Geometry check sheet. Reference: the model listing, model coordinates, mm. Round coordinates to 2 decimals unless told otherwise and drop trailing zeros. Order: outer loops, then holes, each group sorted by start corner. A loop starts at its lowest first (then second) coordinate and runs counter-clockwise, first axis right, second up. Notation, with made-up numbers: M 88.25,19.5 L 92.25,19.5 A27 cw 92.25,35.5 Z; hole C -19,89 d11. An arc over 180 degrees is marked long. Answer as a JSON object with one key per item and string values. Group by question number.
```python
from build123d import *

# Parameters (mm, degrees)
SKETCH_W            = 603
SKETCH_H            = 451
SKETCH_W_2          = 601
SKETCH_H_2          = 449
PAD_DEPTH           = 17
SKETCH001_W         = 603
SKETCH001_H         = 451
PAD001_DEPTH        = 1
LINEARPATTERN_COUNT = 2
LINEARPATTERN_PITCH = 18


with BuildPart() as part:
    # Sketch → Pad (new body)
    with BuildSketch(Plane.XY):
        with Locations((301.5, 225.5)):
            Rectangle(SKETCH_W, SKETCH_H)
        with Locations((301.5, 225.5)):
            Rectangle(SKETCH_W_2, SKETCH_H_2, mode=Mode.SUBTRACT)
    extrude(amount=PAD_DEPTH)

    # Sketch001 (on Face10 of Pad) → Pad001 (join)
    with BuildSketch(Plane.XY.offset(17)):
        with Locations((301.5, 225.5)):
            Rectangle(SKETCH001_W, SKETCH001_H)
        Polygon((22.025087, 14), (179.143913, 14), (100.981365, 101.689824), align=None, mode=Mode.SUBTRACT)
        Polygon((589, 32.810618), (589, 199.49019), (513.960487, 116.150433), align=None, mode=Mode.SUBTRACT)
        Polygon((585.05717, 437), (427.601062, 437), (505.123787, 348.224991), align=None, mode=Mode.SUBTRACT)
        Polygon((14, 418.188846), (14, 251.509909), (89.039227, 334.849407), align=None, mode=Mode.SUBTRACT)
        Polygon((15.901213, 437), (98.458656, 345.310742), (181.016042, 437), align=None, mode=Mode.SUBTRACT)
        Polygon((225.066216, 437), (304.561693, 348.711335), (384.05717, 437), align=None, mode=Mode.SUBTRACT)
        Polygon((199.854901, 437), (107.878089, 334.84941), (199.979256, 232.560781), (295.142264, 338.25), (206.227357, 437), align=None, mode=Mode.SUBTRACT)
        Polygon((409.014436, 437), (495.688193, 337.745703), (405.061693, 237.094787), (313.981123, 338.25), (402.896029, 437), align=None, mode=Mode.SUBTRACT)
        Polygon((589, 220.412852), (504.541058, 126.611768), (414.481123, 226.633451), (504.96341, 327.124204), (589, 230.889854), align=None, mode=Mode.SUBTRACT)
        Polygon((421.983753, 14), (504.541055, 105.689101), (587.098299, 14), align=None, mode=Mode.SUBTRACT)
        Polygon((223.025087, 14), (300.479294, 100.021605), (377.933555, 14), align=None, mode=Mode.SUBTRACT)
        Polygon((197.898215, 14), (204.186228, 14), (291.059861, 110.482936), (199.979259, 211.638114), (110.405888, 112.156815), align=None, mode=Mode.SUBTRACT)
        Polygon((396.77242, 14), (403.144888, 14), (495.121626, 116.150436), (405.061693, 216.172116), (309.898723, 110.48294), align=None, mode=Mode.SUBTRACT)
        Polygon((14, 220.313669), (101.034043, 122.670999), (190.559826, 222.099446), (98.458659, 324.388075), (14, 230.587239), align=None, mode=Mode.SUBTRACT)
        Polygon((14, 199.273395), (91.609521, 112.204007), (14, 26.009909), align=None, mode=Mode.SUBTRACT)
        Polygon((304.561693, 327.788665), (395.642264, 226.633451), (300.479291, 120.944271), (209.398688, 222.099449), align=None, mode=Mode.SUBTRACT)
        Polygon((514.399004, 337.603492), (589, 252.174295), (589, 420.456285), align=None, mode=Mode.SUBTRACT)
    pad001 = extrude(amount=PAD001_DEPTH)

    # LinearPattern: Pad001 ×2
    with Locations(*[(0, 0, -i * LINEARPATTERN_PITCH) for i in range(1, LINEARPATTERN_COUNT)]):
        add(pad001)


solid = part.part
```
1) Go/stop test with a flat-tipped pin: P1, Ø0.8, axis at x = 344, z = -0.5, coming from the -Y side. Record where the tip stops, or that it passes through.
2) Release check for a two-part mould opening along Y. For faces 1 (the flat face through (460.142, 175.922, -0.507)), 2 (the flat face through (0, 222, 8)) record: +Y half, -Y half, draft (parallel to the pull), parting line (faces both ways), or undercut.
3) Sectioned sample at A-A (z = 12.5). Record the boundary of the cut face in (x, y), then the cut area to 3 significant figures.
4) Thickness scan on line 1 along X through (y, z) = (383.5, 15.25); line 2 along Y through (x, z) = (390, 7); line 3 along Z through (x, y) = (325, 308). Record the ranges inside material, lowest first. Write a range as [from, to].
5) Sectioned sample at B-B (y = 57). Count the separate pieces of the cut face and the enclosed holes in it, then the cut area to 3 significant figures.
Final values:
{
 "1": {"P1": "stops at y = 0"},
 "2": {"face 1": "undercut", "face 2": "draft"},
 "3": {"outline": "M 0,0 L 603,0 L 603,451 L 0,451 Z; hole M 1,1 L 602,1 L 602,450 L 1,450 Z", "area": "2,100 mm^2"},
 "4": {"line 1": "x = [0, 1], [602, 603]", "line 2": "y = [0, 1], [450, 451]", "line 3": "z = [-1, 0], [17, 18]"},
 "5": {"separate pieces": "14", "enclosed holes": "0", "area": "316 mm^2"}
}
